Model file for the job. Use its own axes, mm. A direction names the side the tool comes from. Give positions to 0.01 mm unless a question says otherwise; leave off trailing zeros. Order: outer loops, then holes, each group sorted by start corner. A loop starts at its lowest first (then second) coordinate and runs counter-clockwise, first axis right, second up. Notation, with made-up numbers: (75, -16) - (94, -16) arc R21 ccw to (94, -4) - close; hole circle Ø11 at (-23, 28). An arc over 180 degrees is marked (long way). Use CSV: the item, a comma, the result in double quotes. Start each with the question number.
(1) Band-saw the part on B-B, the plane y = 18. Give the cut face in (x, z), then the cut area to 3 significant figures.
(2) Band-saw the part on C-C, the plane z = 47. Give the cut face in (x, y), then the cut area to 3 significant figures.
(3) Tool access for faces 4 (the flat face through (13, 20, 80.466)), 5 (the flat face through (13, 20, 0)): list every direction of +Z, -Z, +X, -X, +Y, -Y with a clear straight run to the whole face (end or side of a thin tool).
(4) Drop a flat-ended pin along its axis: pin 1 Ø5 at (y, z) = (5.5, 48.5) entering from -X. Give the stop position or say it passes through.
(5) Band-saw the part on A-A, the plane x = 8. Give the cut face in (y, z).
(6) Probe L1, parallel to Z at x = 9, y = 30.5; L2, parallel to X at y = 10, z = 5. List the from-to ranges inside material, lowest first.
(7) Pull direction Z, two halves, no side cores. Call faces 1 (the flat face through (29, 40, 40)), 2 (the flat face through (14, 20, 79.766)), 3 (the cylindrical face through (28.92, 19.72, 80.06)): +Z half, -Z half, draft (parallel to the pull), parting line (faces both ways), or undercut.
from build123d import *

# Parameters (mm, degrees)
SKETCH1_W              = 140
SKETCH1_H              = 40
BASE_FLANGE1_DEPTH     = 0.7
SKETCHED_BEND1_DEPTH   = 40
SKETCHED_BEND1_2_DEPTH = 40


# Read off the part's stored shape, not the designer's step: Sketched Bend1
# Sheet-metal steps are written as plain solids
with BuildPart() as part:
    # Sketch1 → Base-Flange1 (new body)
    with BuildSketch(Plane.XY):
        with Locations((68.773006135, 20)):
            Rectangle(SKETCH1_W, SKETCH1_H)
    extrude(amount=-BASE_FLANGE1_DEPTH)

    # Sketched Bend1 outline → Sketched Bend1 (cut)
    with BuildSketch(Plane(origin=(0, 0, 0), x_dir=(1, 0, 0), z_dir=(0, 1, 0))):
        with BuildLine():
            ThreePointArc((27.919592491, 0.7), (28.628683458, 0.512803681), (29.152978075, 0))
            Line((29.152978075, 0), (138.773006135, 0))
            Line((138.773006135, 0), (138.773006135, 0.7))
            Line((138.773006135, 0.7), (27.919592491, 0.7))
        make_face()
    extrude(amount=SKETCHED_BEND1_DEPTH, mode=Mode.SUBTRACT)

    # Sketched Bend1 2 outline → Sketched Bend1 2 (add)
    with BuildSketch(Plane(origin=(0, 0, 0), x_dir=(1, 0, 0), z_dir=(0, 1, 0))):
        with BuildLine():
            ThreePointArc((27.919592491, 0), (28.440447346, -0.215745145), (28.656192491, -0.7366))
            Line((28.656192491, -0.7366), (28.656192491, -79.029772711))
            ThreePointArc((28.656192491, -79.029772711), (28.440447346, -79.550627566), (27.919592491, -79.766372711))
            Line((27.919592491, -79.766372711), (-1.226993865, -79.766372711))
            Line((-1.226993865, -79.766372711), (-1.226993865, -80.466372711))
            Line((-1.226993865, -80.466372711), (27.919592491, -80.466372711))
            ThreePointArc((27.919592491, -80.466372711), (28.935422092, -80.045602313), (29.356192491, -79.029772711))
            Line((29.356192491, -79.029772711), (29.356192491, -0.7366))
            ThreePointArc((29.356192491, -0.7366), (29.304457338, -0.354541216), (29.152978075, 0))
            Line((29.152978075, 0), (27.919592491, 0))
        make_face()
    extrude(amount=SKETCHED_BEND1_2_DEPTH)


solid = part.part
Answer block:
1,outline,"(-1.23, -0.7) - (27.92, -0.7) arc R1.44 ccw to (29.36, 0.74) - (29.36, 79.03) arc R1.44 ccw to (27.92, 80.47) - (-1.23, 80.47) - (-1.23, 79.77) - (27.92, 79.77) arc R0.74 cw to (28.66, 79.03) - (28.66, 0.74) arc R0.74 cw to (27.92, 0) - (-1.23, 0) - close"
1,area,"98.0 mm2"
2,outline,"(28.66, 0) - (29.36, 0) - (29.36, 40) - (28.66, 40) - close"
2,area,"28.0 mm2"
3,face 4,"+Z, +X, -X, +Y, -Y"
3,face 5,"-X, +Y, -Y"
4,pin 1,"stops at x = 28.66"
5,outline,"(0, -0.7) - (40, -0.7) - (40, 0) - (0, 0) - close; (0, 79.77) - (40, 79.77) - (40, 80.47) - (0, 80.47) - close"
6,L1,"z = -0.7 to 0, 79.77 to 80.47"
6,L2,"x = 28.66 to 29.36"
7,face 1,"draft"
7,face 2,"undercut"
7,face 3,"+Z half"
